Geometry: see drawing. Coordinates: mm, zero at the bounding-box minimum. A direction names the side the tool comes from. Coordinates: 2 decimals unless noted, no trailing zeros. Write each loop counter-clockwise with the first axis right and the second up, starting at its lowest first coordinate (ties: lowest second). Pieces come first, ordered by that corner, then holes.
1) Pin query (flat end, axial travel): pin 1 Ø6 at (y, z) = (8.5, 14.5) entering from -X; pin 2 Ø5.5 at (x, y) = (16.24, 5.6) entering from +Z; pin 3 Ø4.5 at (y, z) = (14, 13) entering from +X; pin 4 Ø1.5 at (y, z) = (13.5, 3.5) entering from -X. Return the tip coordinate at first contact, or that it passes through.
2) Section query A-A (x = 13). Output: boundary loops of the cut face in (y, z), then the cut area to 3 significant figures.
3) Section query B-B (y = 9.04). Output: boundary loops of the cut face in (x, z), then the cut area to 3 significant figures.
4) Set-up query: the marked faces 1, 2 and 3. Return all of +Z, -Z, +X, -X, +Y, -Y with unobstructed straight access to the full face (end or side cutting, diameter ignored); none if empty.
5) Line query: L1, parallel to Y at x = 13, z = 12.75; L2, parallel to Y at x = 16.24, z = 8; L3, parallel to Y at x = 12.5, z = 14.25. Output: solid intervals per line, ascending.
6) Section query C-C (z = 16.25). Output: boundary loops of the cut face in (x, y).
7) Section query D-D (y = 5.6). Output: boundary loops of the cut face in (x, z).
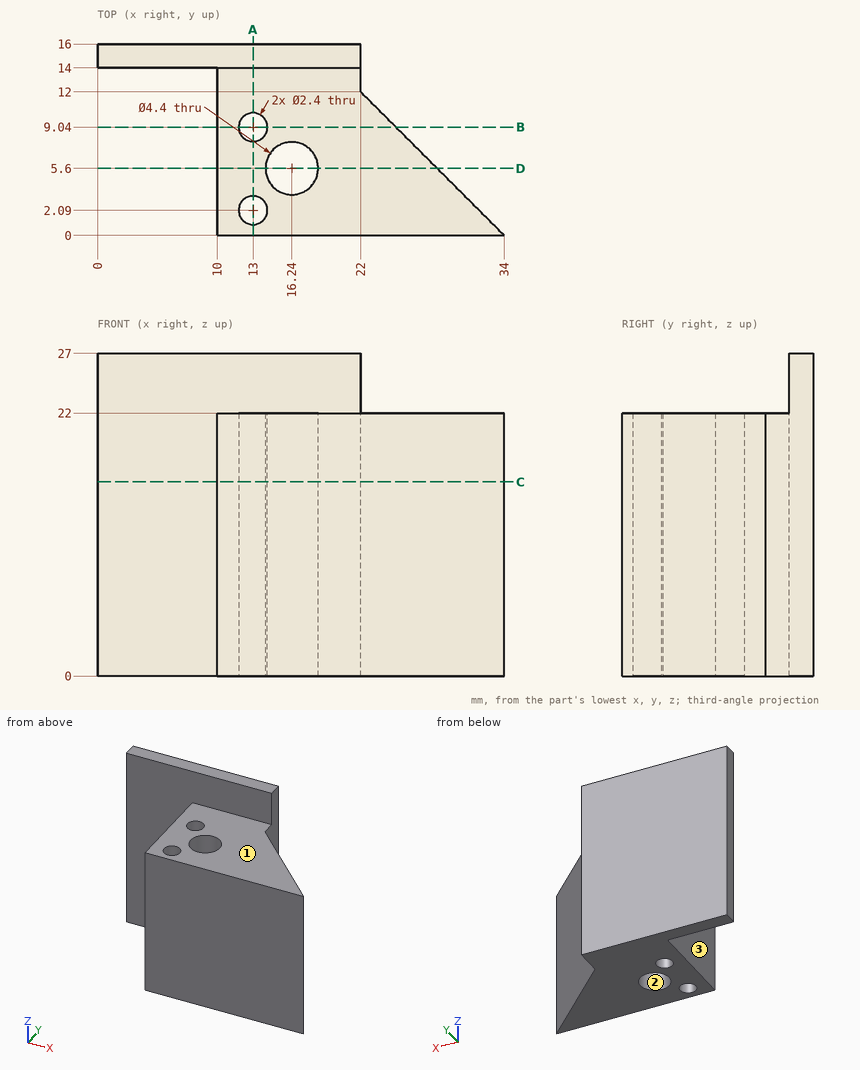
Answer:
1. pin 1: stops at x = 10
1. pin 2: stops at z = 22
1. pin 3: stops at x = 22.25
1. pin 4: stops at x = 0
2. outline: (0, 0) - (0.89, 0) - (0.89, 22) - (0, 22) - close; (3.29, 0) - (7.84, 0) - (7.84, 22) - (3.29, 22) - close; (10.24, 0) - (16, 0) - (16, 27) - (14, 27) - (14, 22) - (10.24, 22) - close
2. area: 256 mm2
3. outline: (10, 0) - (11.8, 0) - (11.8, 22) - (10, 22) - close; (14.2, 0) - (24.96, 0) - (24.96, 22) - (14.2, 22) - close
3. area: 276 mm2
4. face 1: +Z, +X, -X, -Y
4. face 2: +Z, -Z
4. face 3: +Z, -Z, -X, -Y
5. L1: y = 0 to 0.89, 3.29 to 7.84, 10.24 to 16
5. L2: y = 0 to 3.4, 7.8 to 16
5. L3: y = 0 to 1, 3.18 to 7.95, 10.13 to 16
6. outline: (0, 14) - (10, 14) - (10, 0) - (34, 0) - (22, 12) - (22, 16) - (0, 16) - close; hole circle Ø2.4 at (13, 2.09); hole circle Ø2.4 at (13, 9.04); hole circle Ø4.4 at (16.24, 5.6)
7. outline: (10, 0) - (14.04, 0) - (14.04, 22) - (10, 22) - close; (18.44, 0) - (28.4, 0) - (28.4, 22) - (18.44, 22) - close
